Work out the finished part from the listing and answer in its coordinate system (mm). A direction names the side the tool comes from. Coordinates: 2 decimals unless noted, no trailing zeros. Order: outer loops, then holes, each group sorted by start corner. A loop starts at its lowest first (then second) coordinate and runs counter-clockwise, first axis right, second up.
1. Find the intervals of material crossed by probe 1 along Y at (x, z) = (4.5, 4); probe 2 along Z at (x, y) = (-9.5, 0.25); probe 3 along Z at (x, y) = (-41.5, -0.5), in increasing order.
2. The part is cut by section C-C, the plane x = -39. Give the vertices of the cut face in (y, z), then the cut area to 3 significant figures.
3. A tool of negligible diameter and unlimited length cuts with its end or side. For faces 1 (the cylindrical face through (-31.69, 5.3, -1.67)), 2 (the cylindrical face through (31.17, 5.3, -1.67)), 3 (the cylindrical face through (-0.17, -1.38, 6.2)), from which of +Z, -Z, +X, -X, +Y, -Y can it reach the whole face along a straight path? Write none if from no direction.
4. Flat-ended cylindrical pins translate along their axes: pin 1 Ø2 at (x, z) = (31.5, -5) entering from -Y; pin 2 Ø1.5 at (x, y) = (-12.5, -3.5) entering from +Z; pin 3 Ø2 at (x, z) = (8.5, 4.5) entering from +Y; pin 4 Ø2 at (y, z) = (4.5, 3) entering from +X. Find the tip coordinate at first contact, or state that the pin passes through.
5. The part is cut by section D-D, the plane x = 2. Give the vertices of the cut face in (y, z), then the cut area to 3 significant figures.
```python
from build123d import *

# Parameters (mm, degrees)
CHAMFER1_SIZE = 0.635


with BuildPart() as part:
    # Sketch1 → Revolve1 (revolve)
    with BuildSketch(Plane.XY):
        with BuildLine():
            Line((-50.8, 0), (50.8, 0))
            Line((50.8, 0), (50.8, 5.55625))
            Line((50.8, 5.55625), (12.7, 5.55625))
            ThreePointArc((12.7, 5.55625), (12.138733992, 5.788733992), (11.90625, 6.35))
            Line((11.90625, 6.35), (-11.90625, 6.35))
            ThreePointArc((-11.90625, 6.35), (-12.138733992, 5.788733992), (-12.7, 5.55625))
            Line((-12.7, 5.55625), (-50.8, 5.55625))
            Line((-50.8, 5.55625), (-50.8, 0))
        make_face()
    revolve(axis=Axis((-50.8, 0, 0), (-1, 0, 0)))

    # Chamfer1
    chamfer1_edges = [part.edges().sort_by_distance(p)[0] for p in [
        (-50.8, -5.55625, 0),
        (50.8, -5.55625, 0),
    ]]
    chamfer(chamfer1_edges, length=CHAMFER1_SIZE)


solid = part.part
```
Geometry says:
1. probe 1: y = -4.93 to 4.93
1. probe 2: z = -6.35 to 6.35
1. probe 3: z = -5.53 to 5.53
2. outline: circle Ø11.11 at (0, 0)
2. area: 97.0 mm2
3. face 1: -X
3. face 2: +X
3. face 3: +X, -X
4. pin 1: stops at y = -3.86
4. pin 2: stops at z = 5.57
4. pin 3: stops at y = 5.3
4. pin 4: stops at x = 50.8
5. outline: circle Ø12.7 at (0, 0)
5. area: 127 mm2
